```python
from build123d import *

# Parameters (mm, degrees)
SKETCH1_R           = 1.47
BOSS_EXTRUDE1_DEPTH = 1.5875


with BuildPart() as part:
    # Sketch1 → Boss-Extrude1 (new, symmetric)
    with BuildSketch(Plane.XY):
        Polygon((-12.5, 35), (-60, 35), (-60, 12.5), (-63.175, 12.5), (-63.175, -12.5), (-60, -12.5), (-60, -35), (-12.5, -35), (-12.5, -31.825), (-1.47, -31.825), (-1.47, -28.125), (-3.25, -28.125), (-3.25, -25.525), (-1.47, -25.525), (-1.47, -21.825), (1.47, -21.825), (1.47, -25.525), (3.25, -25.525), (3.25, -28.125), (1.47, -28.125), (1.47, -31.825), (12.5, -31.825), (12.5, -35), (60, -35), (60, -12.5), (63.175, -12.5), (63.175, 12.5), (60, 12.5), (60, 35), (12.5, 35), (12.5, 31.825), (1.47, 31.825), (1.47, 28.125), (3.25, 28.125), (3.25, 25.525), (1.47, 25.525), (1.47, 21.825), (-1.47, 21.825), (-1.47, 25.525), (-3.25, 25.525), (-3.25, 28.125), (-1.47, 28.125), (-1.47, 31.825), (-12.5, 31.825), align=None)
        with Locations((-61.5875, 0)):
            Circle(SKETCH1_R, mode=Mode.SUBTRACT)
        with Locations(Location((61.5875, 0, 0), (0, 0, 180))):
            Circle(SKETCH1_R, mode=Mode.SUBTRACT)
    extrude(amount=BOSS_EXTRUDE1_DEPTH, both=True)


solid = part.part
```
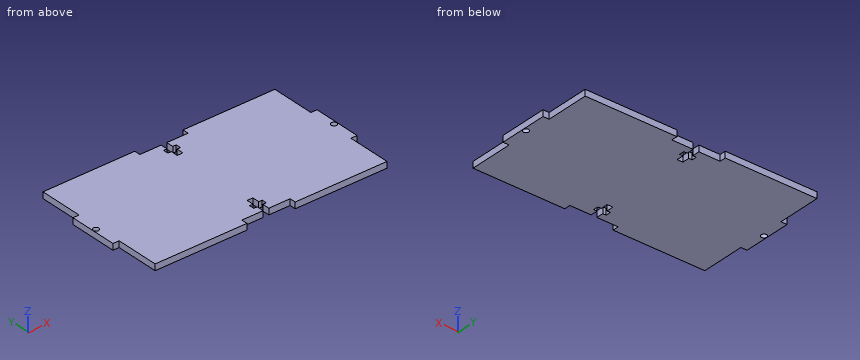
Geometry: final body of the model. Coordinates: model frame, mm. Round coordinates to 2 decimals unless told otherwise and drop trailing zeros. Order: outer loops, then holes, each group sorted by start corner. A loop starts at its lowest first (then second) coordinate and runs counter-clockwise, first axis right, second up. Notation, with made-up numbers: (51.5, 27.25) -> (61.5, 27.25) arc R20 cw to (61.5, 57.25) -> close; hole circle Ø9 at (56.5, -7). An arc over 180 degrees is marked (long way). Use one line per item in the form item = value. Start each with the question number.
1. Cut plane C-C (y = 15.5). Return the cut outline in (x, z), then the cut area to 3 significant figures.
2. Cut plane A-A (y = 0). Count the separate pieces of the cut face and the enclosed holes in it, then the cut area to 3 significant figures.
3. Pin query (flat end, axial travel): pin 1 Ø1 at (y, z) = (26, -0.5) entering from -X; pin 2 Ø1 at (x, z) = (9.5, 0) entering from -Y (3 decimals); pin 3 Ø1.3 at (y, z) = (27, 0) entering from +X. Return the tip coordinate at first contact, or that it passes through.
4. Line query: probe 1 along Y at (x, z) = (2.5, -0.1) (3 decimals); probe 2 along X at (y, z) = (31.5, -0.3); probe 3 along Y at (x, z) = (-0.5, -0.25) (3 decimals). Output: solid intervals per line, ascending.
Solution:
q1.outline = (-60, -1.59) -> (60, -1.59) -> (60, 1.59) -> (-60, 1.59) -> close
q1.area = 381 mm^2
q2.separate_pieces = 3
q2.enclosed_holes = 0
q2.area = 382 mm^2
q3.pin_1 = -60
q3.pin_2 = -31.825
q3.pin_3 = 60
q4.probe_1 = -31.825 to -28.125, -25.525 to 25.525, 28.125 to 31.825
q4.probe_2 = -60 to -1.47, 1.47 to 60
q4.probe_3 = -21.825 to 21.825
